Here's how the part is built. I have some questions about the finished solid (model axes, mm). Face numbers are marked on the shaded views. A direction names the side the tool comes from. Coordinates: 2 decimals unless noted, no trailing zeros. Write each loop counter-clockwise with the first axis right and the second up, starting at its lowest first coordinate (ties: lowest second). Pieces come first, ordered by that corner, then holes. Notation, with made-up numbers: M 41.5,-12.75 L 57.5,-12.75 A29 cw 57.5,13.25 Z; hole C 54,-1 d7. An arc over 180 degrees is marked long. Use a Markdown table: item, result.
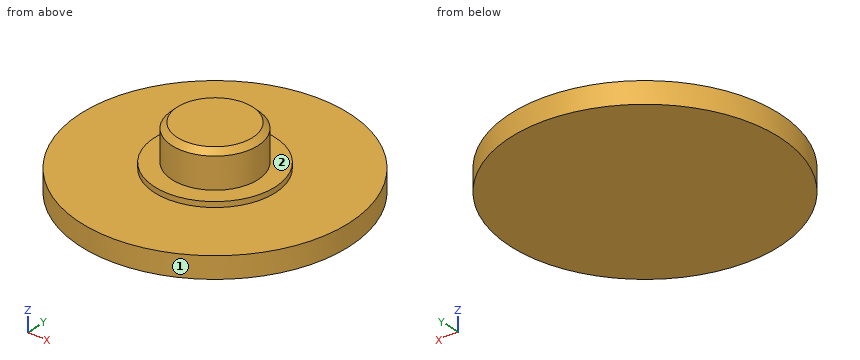
```python
from build123d import *

# Parameters (mm, degrees)
F0_R     = 12.7
F1_DEPTH = 2.032
F2_R     = 4.064
F3_DEPTH = 5.969
F4_SIZE  = 0.508
F5_R     = 5.715
F6_DEPTH = 2.54


with BuildPart() as f1:
    # F0 (on Top) → F1 (new body)
    with BuildSketch(Plane.XY):
        Circle(F0_R)
    extrude(amount=F1_DEPTH)

    # F2 (on Top) → F3 (join)
    with BuildSketch(Plane.XY):
        Circle(F2_R)
    extrude(amount=F3_DEPTH)

    # F4
    f4_edges = [f1.edges().sort_by_distance(p)[0] for p in [
        (-4.064, 0, 5.969),
    ]]
    chamfer(f4_edges, length=F4_SIZE)

    # F5 (on Top) → F6 (join)
    with BuildSketch(Plane.XY):
        Circle(F5_R)
    extrude(amount=F6_DEPTH)


solid = f1.part
```
1. Suppose I cut it at A-A on y = 0. Write out the boundary of the cut face in (x, z) (3 decimals), and give its area (3 significant figures).
Answers follow:
| item | result |
|---|---|
| outline | M -12.7,0 L 12.7,0 L 12.7,2.032 L 5.715,2.032 L 5.715,2.54 L 4.064,2.54 L 4.064,5.461 L 3.556,5.969 L -3.556,5.969 L -4.064,5.461 L -4.064,2.54 L -5.715,2.54 L -5.715,2.032 L -12.7,2.032 Z |
| area | 85.0 mm2 |
2. Suppose I cut it at D-D on z = 1.65. Write out the boundary of the cut face in (x, y), and give its area (3 significant figures).
Answers follow:
| item | result |
|---|---|
| outline | C 0,0 d25.4 |
| area | 507 mm2 |
3. Suppose I cut it at C-C on z = 3.1. Write out the boundary of the cut face in (x, y).
Answers follow:
| item | result |
|---|---|
| outline | C 0,0 d8.13 |
4. I need wall thicknesses on probe 1 along Z at (x, y) = (-5, -4.75); probe 2 along X at (y, z) = (0, 4.4); probe 3 along Z at (x, y) = (0, 5). Which ranges of each line are inside material? Lowest first, please.
Answers follow:
| item | result |
|---|---|
| probe 1 | z = 0 to 2.03 |
| probe 2 | x = -4.06 to 4.06 |
| probe 3 | z = 0 to 2.54 |
5. Will these pins go through, and if not, where does the flat tip stop? pin 1 Ø8 at (x, y) = (-3, -7) entering from +Z; pin 2 Ø5 at (x, y) = (3, -9) entering from +Z.
Answers follow:
| item | result |
|---|---|
| pin 1 | stops at z = 5.91 |
| pin 2 | stops at z = 2.03 |
6. Which directions (+Z, -Z, +X, -X, +Y, -Y) give clear straight access to the entire face, cutting with the end or side of a thin tool? Please do the marked faces 1 and 2.
Answers follow:
| item | result |
|---|---|
| face 1 | +Z, -Z |
| face 2 | +Z |
